from build123d import *

# Parameters (mm, degrees)
SKETCH1_R           = 40
BOSS_EXTRUDE1_DEPTH = 5
SKETCH4_R           = 32.5
BOSS_EXTRUDE2_DEPTH = 1
SKETCH5_R           = 25
BOSS_EXTRUDE3_DEPTH = 7
SKETCH6_R           = 2
SKETCH6_R_2         = 8
CUT_EXTRUDE1_DEPTH  = 59.043087444
SKETCH7_R           = 30
CUT_EXTRUDE2_DEPTH  = 4
SKETCH8_R           = 24
CUT_EXTRUDE3_DEPTH  = 4
SKETCH9_R           = 3.61
CUT_EXTRUDE4_DEPTH  = 4
SKETCH10_R          = 1.57
CUT_EXTRUDE5_DEPTH  = 59.043087444
SKETCH11_R          = 2.84
CUT_EXTRUDE6_DEPTH  = 4
SKETCH12_R          = 1.5
CUT_EXTRUDE7_DEPTH  = 4
CUT_EXTRUDE9_DEPTH  = 7
CUT_EXTRUDE10_DEPTH = 4


with BuildPart() as part:
    # Sketch1 → Boss-Extrude1 (new body)
    with BuildSketch(Plane(origin=(0, 0, 0), x_dir=(1, 0, 0), z_dir=(0, 1, 0))):
        with Locations(Location((0, 0, 0), (0, 0, 270))):
            Circle(SKETCH1_R)
    extrude(amount=BOSS_EXTRUDE1_DEPTH)

    # Sketch4 → Boss-Extrude2 (add)
    with BuildSketch(Plane(origin=(0, 5, 0), x_dir=(1, 0, 0), z_dir=(0, 1, 0))):
        with Locations(Location((0, 0, 0), (0, 0, 270))):
            Circle(SKETCH4_R)
    extrude(amount=BOSS_EXTRUDE2_DEPTH)

    # Sketch5 → Boss-Extrude3 (add)
    with BuildSketch(Plane(origin=(0, 6, 0), x_dir=(1, 0, 0), z_dir=(0, 1, 0))):
        with Locations(Location((0, 0, 0), (0, 0, 270))):
            Circle(SKETCH5_R)
    extrude(amount=BOSS_EXTRUDE3_DEPTH)

    # Sketch6 → Cut-Extrude1 (cut, through all)
    with BuildSketch(Plane(origin=(0, 13, 0), x_dir=(1, 0, 0), z_dir=(0, 1, 0))):
        with Locations(Location((12.25, 0, 0), (0, 0, 270))):
            Circle(SKETCH6_R)
        with Locations(Location((0, -12.25, 0), (0, 0, 270))):
            Circle(SKETCH6_R)
        with Locations(Location((-12.25, 0, 0), (0, 0, 270))):
            Circle(SKETCH6_R)
        with Locations(Location((0, 12.25, 0), (0, 0, 270))):
            Circle(SKETCH6_R)
        with Locations(Location((0, 0, 0), (0, 0, 270))):
            Circle(SKETCH6_R_2)
    extrude(amount=-CUT_EXTRUDE1_DEPTH, mode=Mode.SUBTRACT)

    # Sketch7 → Cut-Extrude2 (cut)
    with BuildSketch(Plane.XZ):
        with Locations(Location((0, 0, 0), (0, 0, 270))):
            Circle(SKETCH7_R)
    extrude(amount=-CUT_EXTRUDE2_DEPTH, mode=Mode.SUBTRACT)

    # Sketch8 → Cut-Extrude3 (cut)
    with BuildSketch(Plane.XZ.offset(-4)):
        with Locations(Location((0, 0, 0), (0, 0, 270))):
            Circle(SKETCH8_R)
    extrude(amount=-CUT_EXTRUDE3_DEPTH, mode=Mode.SUBTRACT)

    # Sketch9 → Cut-Extrude4 (cut)
    with BuildSketch(Plane(origin=(0, 13, 0), x_dir=(1, 0, 0), z_dir=(0, 1, 0))):
        with Locations(Location((0, 12.25, 0), (0, 0, 270))):
            Circle(SKETCH9_R)
        with Locations(Location((12.25, 0, 0), (0, 0, 270))):
            Circle(SKETCH9_R)
        with Locations(Location((0, -12.25, 0), (0, 0, 270))):
            Circle(SKETCH9_R)
        with Locations(Location((-12.25, 0, 0), (0, 0, 270))):
            Circle(SKETCH9_R)
    extrude(amount=-CUT_EXTRUDE4_DEPTH, mode=Mode.SUBTRACT)

    # Sketch10 → Cut-Extrude5 (cut, through all)
    with BuildSketch(Plane(origin=(0, 13, 0), x_dir=(1, 0, 0), z_dir=(0, 1, 0))):
        with Locations(Location((0, 33, 0), (0, 0, 270))):
            Circle(SKETCH10_R)
        with Locations(Location((33, 0, 0), (0, 0, 270))):
            Circle(SKETCH10_R)
        with Locations(Location((0, -33, 0), (0, 0, 270))):
            Circle(SKETCH10_R)
        with Locations(Location((-33, 0, 0), (0, 0, 270))):
            Circle(SKETCH10_R)
    extrude(amount=-CUT_EXTRUDE5_DEPTH, mode=Mode.SUBTRACT)

    # Sketch11 → Cut-Extrude6 (cut)
    with BuildSketch(Plane(origin=(0, 6, 0), x_dir=(1, 0, 0), z_dir=(0, 1, 0))):
        with Locations(Location((0, 33, 0), (0, 0, 270))):
            Circle(SKETCH11_R)
        with Locations(Location((33, 0, 0), (0, 0, 270))):
            Circle(SKETCH11_R)
        with Locations(Location((0, -33, 0), (0, 0, 270))):
            Circle(SKETCH11_R)
        with Locations(Location((-33, 0, 0), (0, 0, 270))):
            Circle(SKETCH11_R)
    extrude(amount=-CUT_EXTRUDE6_DEPTH, mode=Mode.SUBTRACT)

    # Sketch12 → Cut-Extrude7 (cut)
    with BuildSketch(Plane(origin=(0, 13, 0), x_dir=(1, 0, 0), z_dir=(0, 1, 0))):
        with Locations(Location((0, -21.5, 0), (0, 0, 270))):
            Circle(SKETCH12_R)
        with Locations(Location((-15.202795796, -15.202795796, 0), (0, 0, 270))):
            Circle(SKETCH12_R)
        with Locations(Location((-21.5, 0, 0), (0, 0, 270))):
            Circle(SKETCH12_R)
        with Locations(Location((-15.202795796, 15.202795796, 0), (0, 0, 270))):
            Circle(SKETCH12_R)
        with Locations(Location((0, 21.5, 0), (0, 0, 270))):
            Circle(SKETCH12_R)
        with Locations(Location((15.202795796, 15.202795796, 0), (0, 0, 270))):
            Circle(SKETCH12_R)
        with Locations(Location((21.5, 0, 0), (0, 0, 270))):
            Circle(SKETCH12_R)
        with Locations(Location((15.202795796, -15.202795796, 0), (0, 0, 270))):
            Circle(SKETCH12_R)
    extrude(amount=-CUT_EXTRUDE7_DEPTH, mode=Mode.SUBTRACT)

    # Sketch13 → Cut-Extrude9 (cut)
    with BuildSketch(Plane.XZ.offset(-4)):
        Polygon((15.202795796, -11.969634288), (12.402795796, -13.586215042), (12.402795796, -16.819376549), (15.202795796, -18.435957303), (18.002795796, -16.819376549), (18.002795796, -13.586215042), align=None)
        Polygon((-15.202795796, 11.969634288), (-12.402795796, 13.586215042), (-12.402795796, 16.819376549), (-15.202795796, 18.435957303), (-18.002795796, 16.819376549), (-18.002795796, 13.586215042), align=None)
    extrude(amount=-CUT_EXTRUDE9_DEPTH, mode=Mode.SUBTRACT)

    # Sketch14 → Cut-Extrude10 (cut)
    with BuildSketch(Plane.XZ):
        with BuildLine():
            ThreePointArc((-24.74274405, 16.964569457), (-21.213203436, 21.213203436), (-16.964569457, 24.74274405))
            Line((-16.964569457, 24.74274405), (-24.126533346, 31.904707939))
            ThreePointArc((-24.126533346, 31.904707939), (-28.284271247, 28.284271247), (-31.904707939, 24.126533346))
            Line((-31.904707939, 24.126533346), (-24.74274405, 16.964569457))
        make_face()
    extrude(amount=-CUT_EXTRUDE10_DEPTH, mode=Mode.SUBTRACT)


solid = part.part
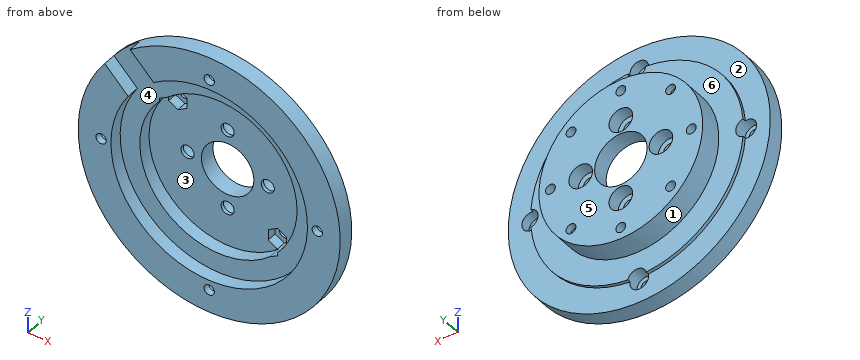
For this review, take the finished solid that the model builds, in its own axes (mm). Face numbers are marked on the shaded views. A direction names the side the tool comes from. Give positions to 0.01 mm unless a question says otherwise; leave off trailing zeros. Loops run counter-clockwise (first coordinate to the right, second up) from the corner with the lowest first, then second, coordinate; pieces in that order, holes last. Notation, with made-up numbers: (14, 89.25) - (56, 89.25) arc R29 cw to (56, 117.25) - close; hole circle Ø1 at (-1.5, -37.75). An arc over 180 degrees is marked (long way). Write each question's results on one line, items separated by ' | '.
(1) Take a section at C-C (z = -21.5). Give the boundary of the cut face in (x, y), then the cut area to 3 significant figures.
Conclusion:
outline: (-33.73, 0) - (-20.92, 0) - (-20.92, 4) - (-10.67, 4) - (-10.67, 8) - (10.67, 8) - (10.67, 4) - (20.92, 4) - (20.92, 0) - (33.73, 0) - (33.73, 5) - (24.37, 5) - (24.37, 6) - (12.76, 6) - (12.76, 13) - (1.5, 13) - (1.5, 9) - (-1.5, 9) - (-1.5, 13) - (-12.76, 13) - (-12.76, 6) - (-24.37, 6) - (-24.37, 5) - (-33.73, 5) - close | area: 300 mm^2
(2) Take a section at D-D (x = 21.5). Give the boundary of the cut face in (y, z).
Conclusion:
outline: (0, -33.73) - (5, -33.73) - (5, -24.37) - (6, -24.37) - (6, -12.76) - (13, -12.76) - (13, -1.5) - (9, -1.5) - (9, 1.5) - (13, 1.5) - (13, 12.76) - (6, 12.76) - (6, 24.37) - (5, 24.37) - (5, 33.73) - (0, 33.73) - (0, 20.92) - (4, 20.92) - (4, 10.67) - (8, 10.67) - (8, -10.67) - (4, -10.67) - (4, -20.92) - (0, -20.92) - close
(3) Take a section at B-B (x = -28). Give the boundary of the cut face in (y, z).
Conclusion:
outline: (0, -28.57) - (5, -28.57) - (5, -16.5) - (6, -16.5) - (6, 16.5) - (5, 16.5) - (5, 28.57) - (4, 28.57) - (4, 20.22) - (0, 20.22) - (0, 10.77) - (4, 10.77) - (4, -10.77) - (0, -10.77) - close
(4) For pin 1 Ø1.5 at (y, z) = (7.5, -10.5) entering from -X; pin 2 Ø3 at (y, z) = (9.5, 19) entering from +X; pin 3 Ø12 at (x, z) = (31, -8.5) entering from +Y; pin 4 Ø2.5 at (x, z) = (0, 12.25) entering from +Y, all flat-tipped, find the tip position at first contact; note any pin that passes through.
Conclusion:
pin 1: x = -23.02 | pin 2: x = 17.85 | pin 3: y = 6 | pin 4: through
(5) For the marked faces 4, 5 and 6, list the 3-axis set-ups (+Z, -Z, +X, -X, +Y, -Y) from which the entire face can be reached by the end or side of a thin tool; tool diameter is ignored.
Conclusion:
face 4: -Y | face 5: +Z, -Z, +X, -X, +Y | face 6: +Y
(6) Take a section at A-A (z = 0). State how many separate pieces and enclosed holes the cut face has, then the cut area to 3 significant figures.
Conclusion:
separate pieces: 6 | enclosed holes: 0 | area: 162 mm^2
(7) Draft analysis for pull direction Z (two halves, no side actions). For the marked faces 1, 2 and 3, state which applies: +Z half, -Z half, draft (parallel to the pull), parting line (faces both ways), or undercut.
Conclusion:
face 1: parting line | face 2: draft | face 3: undercut
(8) For line 1 along Z through (x, y) = (-2, 10); line 2 along Z through (x, y) = (-14.5, 10.5); line 3 along Y through (x, z) = (-28.5, 12), list the stretches that pass through material, from the lowest coordinate up.
Conclusion:
line 1: -24.92 to -15.26, -9.24 to -7.75, 7.75 to 9.24, 15.26 to 24.92 | line 2: -20.37 to -16.53, -13.88 to -2.82, 2.82 to 12.38, 18.03 to 20.37 | line 3: 0 to 6
